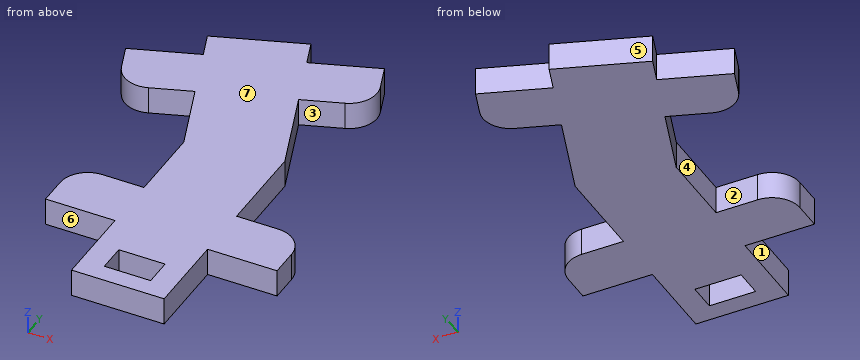
```python
from build123d import *

# Parameters (mm, degrees)
SKETCH1_W           = 5
SKETCH1_H           = 3
BOSS_EXTRUDE1_DEPTH = 3


with BuildPart() as part:
    # Sketch1 → Boss-Extrude1 (new body)
    with BuildSketch(Plane.XY):
        with BuildLine():
            Line((0, -14.236730193), (0, -23.236730193))
            Line((0, -23.236730193), (10, -23.236730193))
            Line((10, -23.236730193), (10, -14.236730193))
            Line((10, -14.236730193), (17.5, -14.236730193))
            Line((17.5, -14.236730193), (17.5, -11.236730193))
            ThreePointArc((17.5, -11.236730193), (16.621320344, -9.115409849), (14.5, -8.236730193))
            Line((14.5, -8.236730193), (10, -8.236730193))
            Line((10, -8.236730193), (10, 1.763269807))
            Line((10, 1.763269807), (6.579798567, 11.160196015))
            Line((6.579798567, 11.160196015), (10.80841536, 12.69928666))
            ThreePointArc((10.80841536, 12.69928666), (12.501278291, 14.250509737), (12.601432793, 16.544424952))
            Line((12.601432793, 16.544424952), (11.575372363, 19.363502815))
            Line((11.575372363, 19.363502815), (4.527677707, 16.79835174))
            Line((4.527677707, 16.79835174), (3.501617277, 19.617429602))
            Line((3.501617277, 19.617429602), (-5.895308931, 16.197228169))
            Line((-5.895308931, 16.197228169), (-4.869248501, 13.378150306))
            Line((-4.869248501, 13.378150306), (-11.916943157, 10.812999231))
            Line((-11.916943157, 10.812999231), (-10.890882727, 7.993921369))
            ThreePointArc((-10.890882727, 7.993921369), (-9.33965965, 6.301058438), (-7.045744435, 6.200903937))
            Line((-7.045744435, 6.200903937), (-2.817127641, 7.739994582))
            Line((-2.817127641, 7.739994582), (0, 0))
            Line((0, 0), (0, -8.236730193))
            Line((0, -8.236730193), (-4.5, -8.236730193))
            ThreePointArc((-4.5, -8.236730193), (-6.621320344, -9.115409849), (-7.5, -11.236730193))
            Line((-7.5, -11.236730193), (-7.5, -14.236730193))
            Line((-7.5, -14.236730193), (0, -14.236730193))
        make_face()
        with Locations((5, -19.736730193)):
            Rectangle(SKETCH1_W, SKETCH1_H, mode=Mode.SUBTRACT)
    extrude(amount=BOSS_EXTRUDE1_DEPTH)


solid = part.part
```
Model file for the job. Use its own axes, mm. Face numbers are marked on the shaded views. A direction names the side the tool comes from. Give positions to 0.01 mm unless a question says otherwise; leave off trailing zeros. Loops run counter-clockwise (first coordinate to the right, second up) from the corner with the lowest first, then second, coordinate; pieces in that order, holes last. Notation, with made-up numbers: (6.25, -20) - (45.25, -20) arc R20 ccw to (45.25, -8) - close; hole circle Ø8 at (30, -19). An arc over 180 degrees is marked (long way). One line per item, written item: value. Start each with the question number.
1. Pin check, flat tips, straight feed: pin 1 (1.5 mm diameter, centred on y = -4, z = 1.5, fed in from +X); pin 2 (1.5 mm diameter, centred on x = 13, z = 2, fed in from -Y); pin 3 (0.9 mm diameter, centred on x = -2.5, z = 2, fed in from +Y). Stop position of each tip, or through.
2. Slice it at C-C (x = 14). List the corners of the cut face in (y, z), plus the area to 3 significant figures.
3. Slice it at D-D (y = -10). List the corners of the cut face in (x, z), plus the area to 3 significant figures.
4. Slice it at B-B (x = -0.75). List the corners of the cut face in (y, z), plus the area to 3 significant figures.
5. Probe L1, parallel to X at y = -20.5, z = 2.7; L2, parallel to X at y = -8, z = 1.3; L3, parallel to Y at x = 11.25, z = 0.7. List the from-to ranges inside material, lowest first. Write a range as from..to.
6. Pull direction Y, two halves, no side cores. Call the marked faces 4, 5, 6 and 7: pulls with the +Y half, pulls with the -Y half, needs draft (parallel to the pull), parting line crosses it, or undercut.
7. Which spindle directions (+Z, -Z, +X, -X, +Y, -Y) get a long thin tool onto all of the face, cutting with end or side? Do the marked faces 1, 2 and 3. Say none if no direction does.
Solution:
1. pin 1: stops at x = 10
1. pin 2: stops at y = -14.24
1. pin 3: stops at y = 17.6
2. outline: (-14.24, 0) - (-8.24, 0) - (-8.24, 3) - (-14.24, 3) - close
2. area: 18.0 mm^2
3. outline: (-7.23, 0) - (17.23, 0) - (17.23, 3) - (-7.23, 3) - close
3. area: 73.4 mm^2
4. outline: (-14.24, 0) - (-8.24, 0) - (-8.24, 3) - (-14.24, 3) - close; (2.06, 0) - (18.07, 0) - (18.07, 3) - (2.06, 3) - close
4. area: 66.0 mm^2
5. L1: x = 0..2.5, 7.5..10
5. L2: x = 0..10
5. L3: y = -14.24..-8.24, 12.9..19.25
6. face 4: undercut
6. face 5: pulls with the +Y half
6. face 6: pulls with the -Y half
6. face 7: needs draft
7. face 1: +Z, -Z, -X, -Y
7. face 2: +Z, -Z, -X
7. face 3: +Z, -Z, +X
